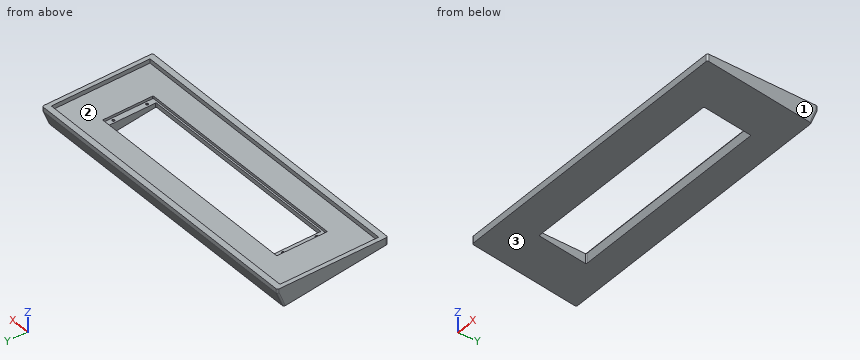
from build123d import *

# Parameters (mm, degrees)
SKETCH3_W                                         = 356.6125
SKETCH3_H                                         = 131.1125
BOSS_EXTRUDE1_DEPTH                               = 5
BOSS_EXTRUDE2_DEPTH                               = 356.6125
SKETCH5_W                                         = 346.6125
SKETCH5_H                                         = 117.1125
CUT_EXTRUDE1_DEPTH                                = 5
SKETCH6_W                                         = 264
SKETCH6_H                                         = 60
CUT_EXTRUDE2_DEPTH                                = 3
SKETCH7_W                                         = 250
SKETCH7_H                                         = 56
CUT_EXTRUDE3_DEPTH                                = 43
FILLET1_R                                         = 1
CSK_FOR_0_FLAT_HEAD_MACHINE_SCREW_100_D           = 1.778
CSK_FOR_0_FLAT_HEAD_MACHINE_SCREW_100_DEPTH       = 5
CSK_FOR_0_FLAT_HEAD_MACHINE_SCREW_100_CSINK_D     = 3.0226
CSK_FOR_0_FLAT_HEAD_MACHINE_SCREW_100_CSINK_ANGLE = 100
CSK_FOR_0_FLAT_HEAD_MACHINE_SCREW_100_TIP         = 0.53416509
CSK_FOR_0_FLAT_HEAD_MACHINE_SCREW_2_D             = 1.778
CSK_FOR_0_FLAT_HEAD_MACHINE_SCREW_2_DEPTH         = 5
CSK_FOR_0_FLAT_HEAD_MACHINE_SCREW_2_CSINK_D       = 3.0226
CSK_FOR_0_FLAT_HEAD_MACHINE_SCREW_2_CSINK_ANGLE   = 100
CSK_FOR_0_FLAT_HEAD_MACHINE_SCREW_2_TIP           = 0.53416509
FILLET2_R                                         = 2


with BuildPart() as part:
    # Sketch3 → Boss-Extrude1 (new body)
    with BuildSketch(Plane.XY):
        with Locations((178.80625, 57.983485256)):
            Rectangle(SKETCH3_W, SKETCH3_H)
    extrude(amount=-BOSS_EXTRUDE1_DEPTH)

    # Sketch4 → Boss-Extrude2 (add)
    with BuildSketch(Plane.ZY.offset(-0.5)):
        Polygon((-5, -7.572764744), (-8.365004472, -7.572764744), (-23.543677091, 116.047603388), (-5, 123.539735256), align=None)
    extrude(amount=-BOSS_EXTRUDE2_DEPTH)

    # Sketch5 → Cut-Extrude1 (cut)
    with BuildSketch(Plane.XY):
        with Locations((178.80625, 57.983485256)):
            Rectangle(SKETCH5_W, SKETCH5_H)
    extrude(amount=-CUT_EXTRUDE1_DEPTH, mode=Mode.SUBTRACT)

    # Sketch6 → Cut-Extrude2 (cut)
    with BuildSketch(Plane.XY.offset(-5)):
        with Locations((178.80625, 57.983485256)):
            Rectangle(SKETCH6_W, SKETCH6_H)
    extrude(amount=-CUT_EXTRUDE2_DEPTH, mode=Mode.SUBTRACT)

    # Sketch7 → Cut-Extrude3 (cut)
    with BuildSketch(Plane.XY.offset(-8)):
        with Locations((178.80625, 57.983485256)):
            Rectangle(SKETCH7_W, SKETCH7_H)
    extrude(amount=-CUT_EXTRUDE3_DEPTH, mode=Mode.SUBTRACT)

    # Fillet1
    fillet1_edges = [part.edges().sort_by_distance(p)[0] for p in [
        (46.80625, 27.983485256, -6.5),
        (46.80625, 87.983485256, -6.5),
        (310.80625, 87.983485256, -6.5),
        (310.80625, 27.983485256, -6.5),
        (53.80625, 29.983485256, -10.488166069),
        (53.80625, 85.983485256, -13.926133774),
        (303.80625, 85.983485256, -13.926133774),
        (303.80625, 29.983485256, -10.488166069),
    ]]
    fillet(fillet1_edges, radius=FILLET1_R)

    # CSK for _0 Flat Head Machine Screw _100
    with Locations(Plane.XY.offset(-8)):
        with Locations((50.30625, 77.983485256), (50.30625, 37.983485256)):
            CounterSinkHole(CSK_FOR_0_FLAT_HEAD_MACHINE_SCREW_100_D / 2, CSK_FOR_0_FLAT_HEAD_MACHINE_SCREW_100_CSINK_D / 2, depth=CSK_FOR_0_FLAT_HEAD_MACHINE_SCREW_100_DEPTH, counter_sink_angle=CSK_FOR_0_FLAT_HEAD_MACHINE_SCREW_100_CSINK_ANGLE)
            with Locations((0, 0, -(CSK_FOR_0_FLAT_HEAD_MACHINE_SCREW_100_DEPTH + CSK_FOR_0_FLAT_HEAD_MACHINE_SCREW_100_TIP / 2))):  # 118° drill point
                Cone(0, CSK_FOR_0_FLAT_HEAD_MACHINE_SCREW_100_D / 2, CSK_FOR_0_FLAT_HEAD_MACHINE_SCREW_100_TIP, mode=Mode.SUBTRACT)

    # CSK for _0 Flat Head Machine Screw _ 2
    with Locations(Plane.XY.offset(-8)):
        with Locations((307.30625, 77.983485256), (307.30625, 37.983485256)):
            CounterSinkHole(CSK_FOR_0_FLAT_HEAD_MACHINE_SCREW_2_D / 2, CSK_FOR_0_FLAT_HEAD_MACHINE_SCREW_2_CSINK_D / 2, depth=CSK_FOR_0_FLAT_HEAD_MACHINE_SCREW_2_DEPTH, counter_sink_angle=CSK_FOR_0_FLAT_HEAD_MACHINE_SCREW_2_CSINK_ANGLE)
            with Locations((0, 0, -(CSK_FOR_0_FLAT_HEAD_MACHINE_SCREW_2_DEPTH + CSK_FOR_0_FLAT_HEAD_MACHINE_SCREW_2_TIP / 2))):  # 118° drill point
                Cone(0, CSK_FOR_0_FLAT_HEAD_MACHINE_SCREW_2_D / 2, CSK_FOR_0_FLAT_HEAD_MACHINE_SCREW_2_TIP, mode=Mode.SUBTRACT)

    # Fillet2
    fillet2_edges = [part.edges().sort_by_distance(p)[0] for p in [
        (0.5, 119.793669322, -14.271838546),
        (357.1125, 119.793669322, -14.271838546),
        (357.1125, -7.572764744, -4.182502236),
        (0.5, -7.572764744, -4.182502236),
        (0.5, 123.539735256, -2.5),
        (357.1125, 123.539735256, -2.5),
    ]]
    fillet(fillet2_edges, radius=FILLET2_R)


solid = part.part
Design review of the part built by this model. Coordinates are the model's own, in mm. Face numbers are marked on the shaded views. Coordinates: 2 decimals unless noted, no trailing zeros. Order: outer loops, then holes, each group sorted by start corner. A loop starts at its lowest first (then second) coordinate and runs counter-clockwise, first axis right, second up.
Item 1: For line 1 (X direction, y = 55.5, z = -3); line 2 (X direction, y = 48, z = -11); line 3 (Y direction, x = 30.5, z = -3.5), list the stretches that pass through material, from the lowest coordinate up.
Item 2: Take a section at C-C, the plane x = 22. Write out the cut boundary in (y, z) (3 decimals), then the cut area to 3 significant figures.
Item 3: For pin 1 Ø2 at (x, y) = (50.31, 77.98) entering from +Z; pin 2 Ø1.5 at (x, z) = (168.5, -6) entering from +Y; pin 3 Ø10 at (x, z) = (310.5, -20.5) entering from +Y, all flat-tipped, find the tip position at first contact; note any pin that passes through.
Item 4: Take a section at D-D, the plane y = 18.5. Write out the cut boundary in (x, z), then the cut area to 3 significant figures.
Item 5: Take a section at A-A, the plane x = 267. Write out the cut boundary in (y, z) (3 decimals).
Item 6: Take a section at B-B, the plane y = 49.5. Write out the cut boundary in (x, z).
Item 7: The part is to be moulded in two halves that separate along Y. For the marked faces 1, 2 and 3, say which applies: pulls with the +Y half, pulls with the -Y half, needs draft (parallel to the pull), parting line crosses it, or undercut.
The answers:
1. line 1: x = 0.5 to 5.5, 352.11 to 357.11
1. line 2: x = 0.5 to 53.81, 303.81 to 357.11
1. line 3: y = -7.57 to -0.57, 116.54 to 123.54
2. outline: (-7.573, -8.365) - (116.048, -23.544) - (123.54, -5) - (123.54, 0) - (116.54, 0) - (116.54, -5) - (-0.573, -5) - (-0.573, 0) - (-7.573, 0) - close
2. area: 1,490 mm2
3. pin 1: stops at z = -8.42
3. pin 2: stops at y = 123.44
3. pin 3: stops at y = 119.3
4. outline: (0.5, -11.57) - (357.11, -11.57) - (357.11, 0) - (352.11, 0) - (352.11, -5) - (5.5, -5) - (5.5, 0) - (0.5, 0) - close
4. area: 2,390 mm2
5. outline: (-7.573, -8.365) - (29.983, -12.976) - (29.983, -8) - (27.983, -8) - (27.983, -5) - (-0.573, -5) - (-0.573, 0) - (-7.573, 0) - close; (85.983, -19.852) - (116.048, -23.544) - (123.54, -5) - (123.54, 0) - (116.54, 0) - (116.54, -5) - (87.983, -5) - (87.983, -8) - (85.983, -8) - close
6. outline: (0.5, -15.37) - (53.81, -15.37) - (53.81, -8) - (46.81, -8) - (46.81, -5) - (5.5, -5) - (5.5, 0) - (0.5, 0) - close; (303.81, -15.37) - (357.11, -15.37) - (357.11, 0) - (352.11, 0) - (352.11, -5) - (310.81, -5) - (310.81, -8) - (303.81, -8) - close
7. face 1: needs draft
7. face 2: undercut
7. face 3: pulls with the -Y half
